from build123d import *

# Parameters (mm, degrees)
F2_DEPTH  = 25
F3_DEPTH  = 25
F10_R     = 3.25
F11_DEPTH = 50
F12_R     = 3.25
F13_DEPTH = 50
F14_R     = 3.25
F15_DEPTH = 120
F22_R     = 3.25
F23_DEPTH = 100
F24_R     = 3.25
F25_DEPTH = 100


with BuildPart() as f2:
    # F1 (on Top) → F2 (new body)
    with BuildSketch(Plane.XY):
        Polygon((-45, -60), (-40, -60), (40, -60), (40, 39.9669196701), (-36.0033019851, 39.9669196701), (-39.0033019851, 39.9669196701), (-42.0016509926, 40.0664346415), (-45, 40.1659496129), align=None)
        Polygon((37, -57), (-37, -57), (-42.0016509926, -57), (-42.0016509926, 37), (-37, 37), (37, 37), align=None, mode=Mode.SUBTRACT)
    extrude(amount=F2_DEPTH)

    # F1 (on Top) → F3 (join)
    with BuildSketch(Plane.XY):
        Polygon((-45, -60), (-40, -60), (40, -60), (40, 39.9669196701), (-36.0033019851, 39.9669196701), (-39.0033019851, 39.9669196701), (-42.0016509926, 40.0664346415), (-45, 40.1659496129), align=None)
        Polygon((37, -57), (-37, -57), (-42.0016509926, -57), (-42.0016509926, 37), (-37, 37), (37, 37), align=None, mode=Mode.SUBTRACT)
    extrude(amount=-F3_DEPTH)

    # F10 (on face) → F11 (cut)
    with BuildSketch(Plane(origin=(8.6602540378, -32.3205080757, 0), x_dir=(-0.9659258263, -0.2588190451, 0), z_dir=(-0.2588190451, 0.9659258263, 0))):
        with Locations((-8.9657547217, 0)):
            Circle(F10_R)
    extrude(amount=-F11_DEPTH, mode=Mode.SUBTRACT)

    # F12 (on face) → F13 (cut)
    with BuildSketch(Plane(origin=(25.9807621135, -15, 0), x_dir=(0.5, 0.8660254038, 0), z_dir=(0.8660254038, -0.5, 0))):
        with Locations((-17.3205080757, 0)):
            Circle(F12_R)
    extrude(amount=F13_DEPTH, mode=Mode.SUBTRACT)

    # F14 (on face) → F15 (cut)
    with BuildSketch(Plane.XZ.offset(60)):
        Circle(F14_R)
    extrude(amount=-F15_DEPTH, mode=Mode.SUBTRACT)

    # F22 (on face) → F23 (cut)
    with BuildSketch(Plane(origin=(1.3397459622, 5, 0), x_dir=(0.9659258263, -0.2588190451, 0), z_dir=(-0.2588190451, -0.9659258263, 0))):
        with Locations((-19.3185165258, 0)):
            Circle(F22_R)
    extrude(amount=F23_DEPTH, mode=Mode.SUBTRACT)

    # F24 (on face) → F25 (cut)
    with BuildSketch(Plane(origin=(-8.6602540378, -5, 0), x_dir=(-0.5, 0.8660254038, 0), z_dir=(0.8660254038, 0.5, 0))):
        with Locations((17.3205080757, 0)):
            Circle(F24_R)
    extrude(amount=-F25_DEPTH, mode=Mode.SUBTRACT)


solid = f2.part
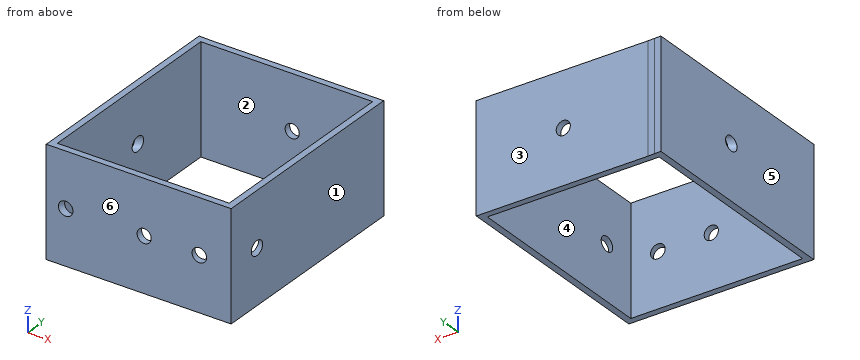
The model under review builds one solid part; all positions refer to its coordinate system, in mm. Face numbers are marked on the shaded views. A direction names the side the tool comes from. Round coordinates to 2 decimals unless told otherwise and drop trailing zeros. Loops run counter-clockwise (first coordinate to the right, second up) from the corner with the lowest first, then second, coordinate; pieces in that order, holes last. Notation, with made-up numbers: (44.5, 31.5) -> (56.5, 31.5) arc R21 ccw to (56.5, 64.5) -> close; hole circle Ø10 at (2.25, 82). An arc over 180 degrees is marked (long way). Write item = value, one per line. Start each with the question number.
Item 1: Insertion check: pin 1 (5 mm diameter, centred on x = 16, z = -18.5, fed in from +Y); pin 2 (6 mm diameter, centred on x = 0, z = 0, fed in from +Y). Each pin has a flat end and moves straight along its axis. Give the tip position at first contact, or say it passes through.
Item 2: Take a section at C-C on z = -13.5. Give the boundary of the cut face in (x, y).
Item 3: Take a section at D-D on x = -29. Give the boundary of the cut face in (y, z), plus the area to 3 significant figures.
Item 4: Mouldability with a two-part tool opening along X and no side actions: class the marked faces 4, 5 and 6 as released by +X, released by -X, zero draft, split by the parting line, or undercut.
Item 5: For the marked faces 1, 2 and 3, list the 3-axis set-ups (+Z, -Z, +X, -X, +Y, -Y) from which the entire face can be reached by the end or side of a thin tool; tool diameter is ignored.
Item 6: To check wall thickness, follow L1, parallel to Y at x = -11, z = -6; L2, parallel to X at y = -11, z = 6; L3, parallel to Z at x = 0, y = -58. State the ranges of each line that lie inside material, in increasing order.
Item 7: Take a section at B-B on x = 0. Give the boundary of the cut face in (y, z).
Item 8: Take a section at A-A on y = -11. Give the boundary of the cut face in (x, z).
Result:
q1.pin_1 = 39.97
q1.pin_2 = through
q2.outline = (-45, -60) -> (40, -60) -> (40, 39.97) -> (-39, 39.97) -> (-45, 40.17) -> close; hole (-42, -57) -> (37, -57) -> (37, 37) -> (-42, 37) -> close
q3.outline = (-60, -25) -> (-57, -25) -> (-57, 25) -> (-60, 25) -> close; (37, -25) -> (39.97, -25) -> (39.97, 25) -> (37, 25) -> close
q3.area = 298 mm²
q4.face_4 = undercut
q4.face_5 = released by -X
q4.face_6 = zero draft
q5.face_1 = +Z, -Z, +X, +Y, -Y
q5.face_2 = +Z, -Z
q5.face_3 = +Z, -Z, +X, +Y
q6.L1 = -60 to -57, 37 to 39.97
q6.L2 = -45 to -42, 37 to 40
q6.L3 = -25 to -3.25, 3.25 to 25
q7.outline = (-60, -25) -> (-57, -25) -> (-57, -3.25) -> (-60, -3.25) -> close; (-60, 3.25) -> (-57, 3.25) -> (-57, 25) -> (-60, 25) -> close; (37, -25) -> (39.97, -25) -> (39.97, -3.25) -> (37, -3.25) -> close; (37, 3.25) -> (39.97, 3.25) -> (39.97, 25) -> (37, 25) -> close
q8.outline = (-45, -25) -> (-42, -25) -> (-42, 25) -> (-45, 25) -> close; (37, -25) -> (40, -25) -> (40, 25) -> (37, 25) -> close
